Part model, mm, in its own coordinate system. Face numbers are marked on the shaded views. Round coordinates to 2 decimals unless told otherwise and drop trailing zeros. Write each loop counter-clockwise with the first axis right and the second up, starting at its lowest first coordinate (ties: lowest second). Pieces come first, ordered by that corner, then holes. Notation, with made-up numbers: M -18.75,86 L 33.25,86 A13 cw 33.25,99 Z; hole C 24,-28.5 d8. An arc over 180 degrees is marked long. One line per question, with ' | ' between items. Start each with the question number.
1) Mould opens along X. For the marked faces 1, 2 and 3 say: pulls with the +X half, pulls with the -X half, needs draft (parallel to the pull), parting line crosses it, or undercut.
2) Saw through at B-B (z = 2.75). List the corners of the cut face in (x, y).
3) Saw through at D-D (x = 2). List the corners of the cut face in (y, z), plus the area to 3 significant figures.
4) Saw through at A-A (x = -13.75). List the corners of the cut face in (y, z), plus the area to 3 significant figures.
5) Saw through at C-C (x = 17). List the corners of the cut face in (y, z).
6) Wall check: probe 1 along X at (y, z) = (0.05, 1.5); probe 2 along Y at (x, z) = (-13.75, 0.45); probe 3 along X at (y, z) = (1.55, 3.4). Give the ranges that are in metal, low to high. Write a range as [from, to].
7) Drop flat-ended pins along their axis: pin 1 Ø2 at (x, y) = (-13.75, 0) entering from +Z; pin 2 Ø1.4 at (x, y) = (18.5, 0) entering from +Z; pin 3 Ø0.5 at (x, z) = (0, 0.5) entering from -Y; pin 4 Ø0.5 at (x, z) = (-15, 0.5) entering from +Y. Give the stop position or say it passes through.
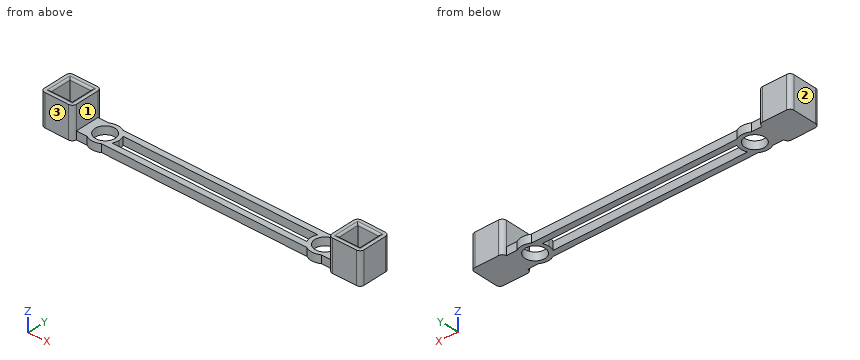
```python
from build123d import *

# Parameters (mm, degrees)
F0_R          = 1.25
F1_DEPTH      = 1
F2_W          = 4
F2_H          = 4
F2_W_2        = 2.7
F2_H_2        = 2.7
F3_DEPTH      = 3
F3_DEPTH_BACK = 1
F4_R          = 0.49999
F5_R          = 0.25


# Not quite as in the source:
# - a fillet or chamfer is up to 0.001 mm smaller than in the source, because OpenCascade refuses the exact size


with BuildPart() as f1:
    # F0 (on Top) → F1 (new body)
    with BuildSketch(Plane.XY):
        with BuildLine():
            Line((0, 0.75), (0, 1.5))
            Line((0, 1.5), (-12.8486121811, 1.5))
            ThreePointArc((-12.8486121811, 1.5), (-12.4533274736, 1.1752192814), (-12.1688611699, 0.75))
            Line((-12.1688611699, 0.75), (0, 0.75))
        make_face()
        with BuildLine():
            ThreePointArc((-12.1688611699, 0.75), (-12.4533274736, 1.1752192814), (-12.8486121811, 1.5))
            Line((-12.8486121811, 1.5), (-14.6513878189, 1.5))
            ThreePointArc((-14.6513878189, 1.5), (-15.5, 0), (-14.6513878189, -1.5))
            Line((-14.6513878189, -1.5), (-12.8486121811, -1.5))
            ThreePointArc((-12.8486121811, -1.5), (-12.4533274736, -1.1752192814), (-12.1688611699, -0.75))
            ThreePointArc((-12.1688611699, -0.75), (-12.0427371391, -0.3843872054), (-12, 0))
            ThreePointArc((-12, 0), (-12.0427371391, 0.3843872054), (-12.1688611699, 0.75))
        make_face()
        with Locations((-13.75, 0)):
            Circle(F0_R, mode=Mode.SUBTRACT)
        with BuildLine():
            Line((-14.6513878189, 1.5), (-12.8486121811, 1.5))
            ThreePointArc((-12.8486121811, 1.5), (-13.75, 1.75), (-14.6513878189, 1.5))
        make_face()
        with BuildLine():
            ThreePointArc((-14.6513878189, -1.5), (-15.5, 0), (-14.6513878189, 1.5))
            Line((-14.6513878189, 1.5), (-19.5, 1.5))
            Line((-19.5, 1.5), (-19.5, -1.5))
            Line((-19.5, -1.5), (-14.6513878189, -1.5))
        make_face()
        with BuildLine():
            Line((-12.8486121811, -1.5), (-14.6513878189, -1.5))
            ThreePointArc((-14.6513878189, -1.5), (-13.75, -1.75), (-12.8486121811, -1.5))
        make_face()
        with BuildLine():
            ThreePointArc((-12.1688611699, -0.75), (-12.4533274736, -1.1752192814), (-12.8486121811, -1.5))
            Line((-12.8486121811, -1.5), (0, -1.5))
            Line((0, -1.5), (0, -0.75))
            Line((0, -0.75), (-12.1688611699, -0.75))
        make_face()
    extrude(amount=F1_DEPTH)

    # F2 (on face) → F3 (join, two sides)
    with BuildSketch(Plane.XY.offset(1)) as f3_sk:
        with Locations((-18, 0)):
            Rectangle(F2_W, F2_H)
        with Locations((-18, 0)):
            Rectangle(F2_W_2, F2_H_2, mode=Mode.SUBTRACT)
    extrude(amount=F3_DEPTH)
    extrude(f3_sk.sketch, amount=-F3_DEPTH_BACK)

    # F4 (radius 0.5 in the source; OpenCascade refuses exactly that, so slightly less here)
    f4_edges = [f1.edges().sort_by_distance(p)[0] for p in [
        (-16, -2, 2),
        (-20, -2, 2),
        (-16, 2, 2),
        (-20, 2, 2),
    ]]
    fillet(f4_edges, radius=F4_R)

    # F5
    f5_edges = [f1.edges().sort_by_distance(p)[0] for p in [
        (-18, -1.35, 4),
        (-16.65, 0, 4),
        (-18, 1.35, 4),
        (-19.35, 0, 4),
    ]]
    fillet(f5_edges, radius=F5_R)

    # F6: F1 across plane


with BuildPart() as f1_1:
    add(f1.part)
    add(f1.part.mirror(Plane.YZ))


solid = f1_1.part
```
Answer key:
1) face 1: undercut | face 2: pulls with the -X half | face 3: needs draft
2) outline: M -20,-1.5 A0.5 ccw -19.5,-2 L -16.5,-2 A0.5 ccw -16,-1.5 L -16,1.5 A0.5 ccw -16.5,2 L -19.5,2 A0.5 ccw -20,1.5 Z; M 16,-1.5 A0.5 ccw 16.5,-2 L 19.5,-2 A0.5 ccw 20,-1.5 L 20,1.5 A0.5 ccw 19.5,2 L 16.5,2 A0.5 ccw 16,1.5 Z; hole M -19.35,-1.35 L -16.65,-1.35 L -16.65,1.35 L -19.35,1.35 Z; hole M 16.65,-1.35 L 19.35,-1.35 L 19.35,1.35 L 16.65,1.35 Z
3) outline: M -1.5,0 L -0.75,0 L -0.75,1 L -1.5,1 Z; M 0.75,0 L 1.5,0 L 1.5,1 L 0.75,1 Z | area: 1.50 mm2
4) outline: M -1.75,0 L -1.25,0 L -1.25,1 L -1.75,1 Z; M 1.25,0 L 1.75,0 L 1.75,1 L 1.25,1 Z | area: 1.00 mm2
5) outline: M -2,0 L 2,0 L 2,4 L 1.6,4 A0.25 ccw 1.35,3.75 L 1.35,1 L -1.35,1 L -1.35,3.75 A0.25 ccw -1.6,4 L -2,4 Z
6) probe 1: x = [-20, -19.35], [-16.65, -16], [16, 16.65], [19.35, 20] | probe 2: y = [-1.75, -1.25], [1.25, 1.75] | probe 3: x = [-20, -16], [16, 20]
7) pin 1: passes through | pin 2: stops at z = 1 | pin 3: stops at y = -1.5 | pin 4: stops at y = 1.5
